Geometry check sheet. Reference: drawing and pictorial views, mm from the part's lowest x, y, z. A direction names the side the tool comes from. Round coordinates to 2 decimals unless told otherwise and drop trailing zeros. Write each loop counter-clockwise with the first axis right and the second up, starting at its lowest first coordinate (ties: lowest second). Pieces come first, ordered by that corner, then holes. Notation, with made-up numbers: M 86,62.25 L 111,62.25 A17 ccw 111,68.25 Z; hole C 74.5,-2 d2. An arc over 180 degrees is marked long. One line per item, written item: value. Start each with the question number.
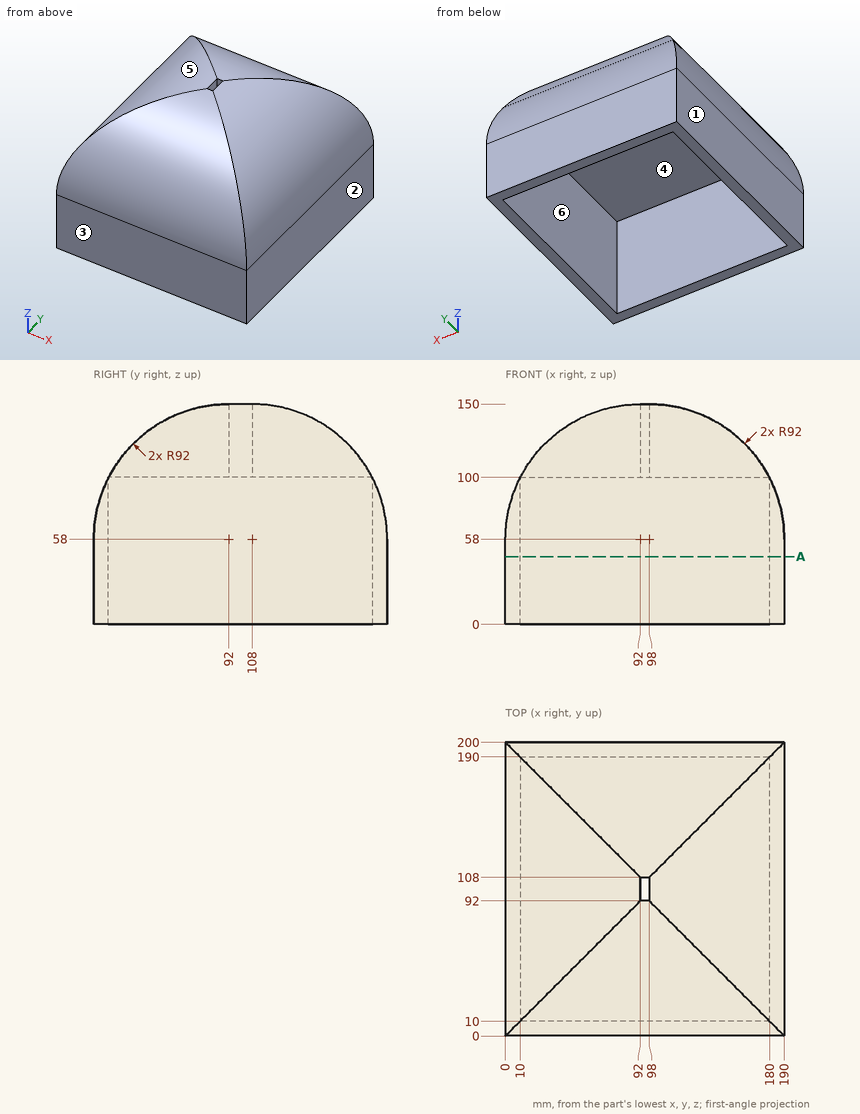
1) Access from +Z, -Z, +X, -X, +Y, -Y to the whole of each face (thin tool, end or side, straight path). Record for the marked faces 5 and 6.
2) Gauge pin test, flat ends, axial feed: pin 1 Ø8 at (x, y) = (20.5, 88.5) entering from -Z; pin 2 Ø1.8 at (x, z) = (96, 123.5) entering from +Y; pin 3 Ø13 at (y, z) = (99.5, 130) entering from -X. Record the tip position at first contact, or that the pin passes through.
3) Thickness scan on line 1 (X direction, y = 46, z = 40); line 2 (Y direction, x = 77.5, z = 13.5); line 3 (Y direction, x = 132, z = 69.5). Record the ranges inside material, lowest first.
4) Mould release check, pull along X, two halves, no side actions. Record for the marked faces 1, 2, 3 and 4: pulls with the +X half, pulls with the -X half, needs draft (parallel to the pull), parting line crosses it, or undercut.
5) Cross-section at A-A (z = 46). Record the boundary of the cut face in (x, y), then the cut area to 3 significant figures.
Results below:
1. face 5: +Z, -X, +Y, -Y
1. face 6: -Z
2. pin 1: stops at z = 100
2. pin 2: stops at y = 173.5
2. pin 3: stops at x = 27.4
3. line 1: x = 0 to 10, 180 to 190
3. line 2: y = 0 to 10, 190 to 200
3. line 3: y = 0.72 to 10, 190 to 199.28
4. face 1: pulls with the -X half
4. face 2: pulls with the +X half
4. face 3: needs draft
4. face 4: undercut
5. outline: M 0,0 L 190,0 L 190,200 L 0,200 Z; hole M 10,10 L 180,10 L 180,190 L 10,190 Z
5. area: 7,400 mm²
